Build history of the part. All positions in model axes, mm. A direction names the side the tool comes from. Give positions to 0.01 mm unless a question says otherwise; leave off trailing zeros. Order: outer loops, then holes, each group sorted by start corner. A loop starts at its lowest first (then second) coordinate and runs counter-clockwise, first axis right, second up. Notation, with made-up numbers: (26.25, -4.75) - (82.25, -4.75) arc R17 cw to (82.25, 4.25) - close; hole circle Ø2 at (4.5, 85). An arc over 180 degrees is marked (long way). Use a Markdown table: item, result. Add a question column.
(1) Slice it at A-A (x = -6). Write the cut outline in (y, z).
(2) Flat gauge pins, fed straight in: pin 1 (12 mm diameter, centred on x = 3.5, y = 29, fed in from +Z); pin 2 (0.9 mm diameter, centred on x = 15.5, y = 2, fed in from +Z); pin 3 (8 mm diameter, centred on x = 16, z = 0, fed in from +Y). Where does each tip first touch, or does it go through?
(3) Wall check: line 1 (X direction, y = 2.25, z = 0); line 2 (X direction, y = 7, z = -1); line 3 (X direction, y = 1.05, z = 20). Give the ranges that are in metal, low to high.
(4) Mould opens along X. For faces 4 (the face through (-10, 1, 20)), 5 (the face through (0, 0, 5)), 6 (the face through (-9.52, 30.73, -8.48)) say: +X half, -X half, draft (parallel to the pull), parting line (faces both ways), or undercut.
(5) Slice it at D-D (z = 20). Write the cut outline in (x, y), then the cut area to 3 significant figures.
(6) Slice it at C-C (x = 0). Write the cut outline in (y, z).
(7) Slice it at B-B (z = 0). Write the cut outline in (x, y), then the cut area to 3 significant figures.
(8) Which spindle directions (+Z, -Z, +X, -X, +Y, -Y) get a long thin tool onto all of the face, cutting with end or side? Do faces 1 (the face through (0, 14, -8)), 2 (the face through (22, 8, -2)), 3 (the face through (10, 1, 20)). Say none if no direction does.
from build123d import *

# Parameters (mm, degrees)
SKETCH1_W           = 50
SKETCH1_H           = 20
BOSS_EXTRUDE1_DEPTH = 3
SKETCH2_W           = 50
SKETCH2_H           = 3
BOSS_EXTRUDE2_DEPTH = 40
CUT_EXTRUDE4_REACH  = 50.218
SKETCH6_R           = 2.5
BOSS_EXTRUDE3_DEPTH = 3
BOSS_EXTRUDE4_DEPTH = 3
SKETCH9_W           = 20
SKETCH9_H           = 3
BOSS_EXTRUDE5_DEPTH = 20
CUT_EXTRUDE5_REACH  = 57.902
SKETCH10_R          = 2.5
SKETCH11_R          = 1.5
CUT_EXTRUDE6_DEPTH  = 3


with BuildPart() as part:
    # Sketch1 → Boss-Extrude1 (new body)
    with BuildSketch(Plane(origin=(0, 0, 0), x_dir=(1, 0, 0), z_dir=(0, 1, 0))):
        Rectangle(SKETCH1_W, SKETCH1_H)
    extrude(amount=BOSS_EXTRUDE1_DEPTH)

    # Sketch2 → Boss-Extrude2 (add)
    with BuildSketch(Plane(origin=(0, 3, 0), x_dir=(1, 0, 0), z_dir=(0, 1, 0))):
        with Locations((0, 8.5)):
            Rectangle(SKETCH2_W, SKETCH2_H)
    extrude(amount=BOSS_EXTRUDE2_DEPTH)

    # Sketch6 → Cut-Extrude4 (cut, up to next)
    with BuildSketch(Plane(origin=(0, 3, 0), x_dir=(1, 0, 0), z_dir=(0, 1, 0)), mode=Mode.PRIVATE) as cut_extrude4_sk1:
        with Locations(Location((-16, 0, 0), (0, 0, 270))):
            Circle(SKETCH6_R)
    cut_extrude4_tool1 = extrude(cut_extrude4_sk1.sketch, amount=-CUT_EXTRUDE4_REACH, mode=Mode.PRIVATE) & part.part
    # Sketch6 → Cut-Extrude4 (cut, up to next)
    with BuildSketch(Plane(origin=(0, 3, 0), x_dir=(1, 0, 0), z_dir=(0, 1, 0)), mode=Mode.PRIVATE) as cut_extrude4_sk2:
        with Locations(Location((16, 0, 0), (0, 0, 270))):
            Circle(SKETCH6_R)
    cut_extrude4_tool2 = extrude(cut_extrude4_sk2.sketch, amount=-CUT_EXTRUDE4_REACH, mode=Mode.PRIVATE) & part.part
    add(cut_extrude4_tool1.solids().sort_by_distance((-16, 3, 0))[0], mode=Mode.SUBTRACT)
    add(cut_extrude4_tool2.solids().sort_by_distance((16, 3, 0))[0], mode=Mode.SUBTRACT)

    # Sketch7 → Boss-Extrude3 (add)
    with BuildSketch(Plane.ZY.offset(25)):
        Polygon((-7, 3), (10, 3), (-7, 20), align=None)
    extrude(amount=-BOSS_EXTRUDE3_DEPTH)

    # Sketch8 → Boss-Extrude4 (add)
    with BuildSketch(Plane(origin=(25, 0, 0), x_dir=(0, 0, -1), z_dir=(1, 0, 0))):
        Polygon((7, 3), (-10, 3), (7, 20), align=None)
    extrude(amount=-BOSS_EXTRUDE4_DEPTH)

    # Sketch9 → Boss-Extrude5 (add)
    with BuildSketch(Plane.XY.offset(10)):
        with Locations((0, 1.5)):
            Rectangle(SKETCH9_W, SKETCH9_H)
    extrude(amount=BOSS_EXTRUDE5_DEPTH)

    # Sketch10 → Cut-Extrude5 (cut, up to next)
    with BuildSketch(Plane(origin=(0, 3, 0), x_dir=(1, 0, 0), z_dir=(0, 1, 0)), mode=Mode.PRIVATE) as cut_extrude5_sk1:
        with Locations(Location((0, -20, 0), (0, 0, 270))):
            Circle(SKETCH10_R)
    cut_extrude5_tool1 = extrude(cut_extrude5_sk1.sketch, amount=-CUT_EXTRUDE5_REACH, mode=Mode.PRIVATE) & part.part
    add(cut_extrude5_tool1.solids().sort_by_distance((0, 3, 20))[0], mode=Mode.SUBTRACT)

    # Sketch11 → Cut-Extrude6 (cut)
    with BuildSketch(Plane.XY.offset(-7)):
        with Locations((9.192388155, 32.192388155)):
            Circle(SKETCH11_R)
        with Locations((9.192388155, 13.807611845)):
            Circle(SKETCH11_R)
        with Locations((-9.192388155, 13.807611845)):
            Circle(SKETCH11_R)
        with Locations((-9.192388155, 32.192388155)):
            Circle(SKETCH11_R)
        with BuildLine():
            Line((15, 43), (25, 43))
            Line((25, 43), (25, 23))
            ThreePointArc((25, 23), (22.360679775, 34.180339887), (15, 43))
        make_face()
        with BuildLine():
            Line((-15, 43), (-25, 43))
            Line((-25, 43), (-25, 23))
            ThreePointArc((-25, 23), (-22.360679775, 34.180339887), (-15, 43))
        make_face()
        with BuildLine():
            Line((-4.358898944, 32), (4.358898944, 32))
            ThreePointArc((4.358898944, 32), (10, 23), (4.358898944, 14))
            Line((4.358898944, 14), (-4.358898944, 14))
            ThreePointArc((-4.358898944, 14), (-10, 23), (-4.358898944, 32))
        make_face()
    extrude(amount=-CUT_EXTRUDE6_DEPTH, mode=Mode.SUBTRACT)


solid = part.part
Solution:
| question | item | result |
|---|---|---|
| 1 | outline | (0, -10) - (15, -10) - (15, -7) - (3, -7) - (3, 30) - (0, 30) - close; (31, -10) - (43, -10) - (43, -7) - (31, -7) - close |
| 2 | pin 1 | z = -7 |
| 2 | pin 2 | z = 10 |
| 2 | pin 3 | y = 3 |
| 3 | line 1 | -25 to -18.5, -13.5 to 13.5, 18.5 to 25 |
| 3 | line 2 | -25 to -22, 22 to 25 |
| 3 | line 3 | -10 to -2.5, 2.5 to 10 |
| 4 | face 4 | -X half |
| 4 | face 5 | draft |
| 4 | face 6 | undercut |
| 5 | outline | (-10, 0) - (-2.5, 0) - (-2.5, 3) - (-10, 3) - close; (2.5, 0) - (10, 0) - (10, 3) - (2.5, 3) - close |
| 5 | area | 45.0 mm2 |
| 6 | outline | (0, -10) - (14, -10) - (14, -7) - (3, -7) - (3, 17.5) - (0, 17.5) - close; (0, 22.5) - (3, 22.5) - (3, 30) - (0, 30) - close; (32, -10) - (43, -10) - (43, -7) - (32, -7) - close |
| 7 | outline | (-25, 0) - (-18.5, 0) - (-18.5, 3) - (-22, 3) - (-22, 13) - (-25, 13) - close; (-13.5, 0) - (13.5, 0) - (13.5, 3) - (-13.5, 3) - close; (18.5, 0) - (25, 0) - (25, 13) - (22, 13) - (22, 3) - (18.5, 3) - close |
| 7 | area | 180 mm2 |
| 8 | face 1 | +Z, -Z |
| 8 | face 2 | +Z, +Y |
| 8 | face 3 | +Z, +X, +Y, -Y |
